from build123d import *

# Parameters (mm, degrees)
BASE_W                        = 80
BASE_H                        = 70
BASE_PLATE_DEPTH              = 3
EXTRUDER_HOLE_CUT_REACH       = 55.235
EXTRUDER_HOLE_R               = 20
EXTRUDER_SREW_HOLES_CUT_REACH = 55.235
EXTRUDER_MOUNT_HOLES_R        = 2.1
LM8_TWO_REACH                 = 55.235
LM8UU_HOLES_R                 = 1.7
LM8_CENTER_REACH              = 55.235
LM8UU_CENTER_R                = 1.7


with BuildPart() as part:
    # Base → Base Plate (new body)
    with BuildSketch(Plane(origin=(0, 0, 0), x_dir=(1, 0, 0), z_dir=(0, 1, 0))):
        Rectangle(BASE_W, BASE_H)
    extrude(amount=BASE_PLATE_DEPTH)

    # Extruder hole → Extruder Hole Cut (cut, up to next)
    with BuildSketch(Plane(origin=(0, 3, 0), x_dir=(1, 0, 0), z_dir=(0, 1, 0)), mode=Mode.PRIVATE) as extruder_hole_cut_sk1:
        with Locations(Location((0, 0, 0), (0, 0, 270))):
            Circle(EXTRUDER_HOLE_R)
    extruder_hole_cut_tool1 = extrude(extruder_hole_cut_sk1.sketch, amount=-EXTRUDER_HOLE_CUT_REACH, mode=Mode.PRIVATE) & part.part
    add(extruder_hole_cut_tool1.solids().sort_by_distance((0, 3, 0))[0], mode=Mode.SUBTRACT)

    # Extruder Mount Holes → Extruder Srew Holes Cut (cut, up to next)
    with BuildSketch(Plane(origin=(0, 3, 0), x_dir=(1, 0, 0), z_dir=(0, 1, 0)), mode=Mode.PRIVATE) as extruder_srew_holes_cut_sk1:
        with Locations(Location((-25, 0, 0), (0, 0, 270))):
            Circle(EXTRUDER_MOUNT_HOLES_R)
    extruder_srew_holes_cut_tool1 = extrude(extruder_srew_holes_cut_sk1.sketch, amount=-EXTRUDER_SREW_HOLES_CUT_REACH, mode=Mode.PRIVATE) & part.part
    # Extruder Mount Holes → Extruder Srew Holes Cut (cut, up to next)
    with BuildSketch(Plane(origin=(0, 3, 0), x_dir=(1, 0, 0), z_dir=(0, 1, 0)), mode=Mode.PRIVATE) as extruder_srew_holes_cut_sk2:
        with Locations(Location((-22.912878475, 10, 0), (0, 0, 270))):
            Circle(EXTRUDER_MOUNT_HOLES_R)
    extruder_srew_holes_cut_tool2 = extrude(extruder_srew_holes_cut_sk2.sketch, amount=-EXTRUDER_SREW_HOLES_CUT_REACH, mode=Mode.PRIVATE) & part.part
    # Extruder Mount Holes → Extruder Srew Holes Cut (cut, up to next)
    with BuildSketch(Plane(origin=(0, 3, 0), x_dir=(1, 0, 0), z_dir=(0, 1, 0)), mode=Mode.PRIVATE) as extruder_srew_holes_cut_sk3:
        with Locations(Location((-22.912878475, -10, 0), (0, 0, 270))):
            Circle(EXTRUDER_MOUNT_HOLES_R)
    extruder_srew_holes_cut_tool3 = extrude(extruder_srew_holes_cut_sk3.sketch, amount=-EXTRUDER_SREW_HOLES_CUT_REACH, mode=Mode.PRIVATE) & part.part
    # Extruder Mount Holes → Extruder Srew Holes Cut (cut, up to next)
    with BuildSketch(Plane(origin=(0, 3, 0), x_dir=(1, 0, 0), z_dir=(0, 1, 0)), mode=Mode.PRIVATE) as extruder_srew_holes_cut_sk4:
        with Locations(Location((25, 0, 0), (0, 0, 270))):
            Circle(EXTRUDER_MOUNT_HOLES_R)
    extruder_srew_holes_cut_tool4 = extrude(extruder_srew_holes_cut_sk4.sketch, amount=-EXTRUDER_SREW_HOLES_CUT_REACH, mode=Mode.PRIVATE) & part.part
    # Extruder Mount Holes → Extruder Srew Holes Cut (cut, up to next)
    with BuildSketch(Plane(origin=(0, 3, 0), x_dir=(1, 0, 0), z_dir=(0, 1, 0)), mode=Mode.PRIVATE) as extruder_srew_holes_cut_sk5:
        with Locations(Location((23, 9.797958971, 0), (0, 0, 270))):
            Circle(EXTRUDER_MOUNT_HOLES_R)
    extruder_srew_holes_cut_tool5 = extrude(extruder_srew_holes_cut_sk5.sketch, amount=-EXTRUDER_SREW_HOLES_CUT_REACH, mode=Mode.PRIVATE) & part.part
    # Extruder Mount Holes → Extruder Srew Holes Cut (cut, up to next)
    with BuildSketch(Plane(origin=(0, 3, 0), x_dir=(1, 0, 0), z_dir=(0, 1, 0)), mode=Mode.PRIVATE) as extruder_srew_holes_cut_sk6:
        with Locations(Location((23, -9.797958971, 0), (0, 0, 270))):
            Circle(EXTRUDER_MOUNT_HOLES_R)
    extruder_srew_holes_cut_tool6 = extrude(extruder_srew_holes_cut_sk6.sketch, amount=-EXTRUDER_SREW_HOLES_CUT_REACH, mode=Mode.PRIVATE) & part.part
    add(extruder_srew_holes_cut_tool1.solids().sort_by_distance((-25, 3, 0))[0], mode=Mode.SUBTRACT)
    add(extruder_srew_holes_cut_tool2.solids().sort_by_distance((-22.912878, 3, -10))[0], mode=Mode.SUBTRACT)
    add(extruder_srew_holes_cut_tool3.solids().sort_by_distance((-22.912878, 3, 10))[0], mode=Mode.SUBTRACT)
    add(extruder_srew_holes_cut_tool4.solids().sort_by_distance((25, 3, 0))[0], mode=Mode.SUBTRACT)
    add(extruder_srew_holes_cut_tool5.solids().sort_by_distance((23, 3, -9.797959))[0], mode=Mode.SUBTRACT)
    add(extruder_srew_holes_cut_tool6.solids().sort_by_distance((23, 3, 9.797959))[0], mode=Mode.SUBTRACT)

    # LM8uu Holes → LM8 Two (cut, up to next)
    with BuildSketch(Plane(origin=(0, 3, 0), x_dir=(1, 0, 0), z_dir=(0, 1, 0)), mode=Mode.PRIVATE) as lm8_two_sk1:
        with Locations(Location((-34, 29, 0), (0, 0, 270))):
            Circle(LM8UU_HOLES_R)
    lm8_two_tool1 = extrude(lm8_two_sk1.sketch, amount=-LM8_TWO_REACH, mode=Mode.PRIVATE) & part.part
    # LM8uu Holes → LM8 Two (cut, up to next)
    with BuildSketch(Plane(origin=(0, 3, 0), x_dir=(1, 0, 0), z_dir=(0, 1, 0)), mode=Mode.PRIVATE) as lm8_two_sk2:
        with Locations(Location((-28, 29, 0), (0, 0, 270))):
            Circle(LM8UU_HOLES_R)
    lm8_two_tool2 = extrude(lm8_two_sk2.sketch, amount=-LM8_TWO_REACH, mode=Mode.PRIVATE) & part.part
    # LM8uu Holes → LM8 Two (cut, up to next)
    with BuildSketch(Plane(origin=(0, 3, 0), x_dir=(1, 0, 0), z_dir=(0, 1, 0)), mode=Mode.PRIVATE) as lm8_two_sk3:
        with Locations(Location((28, 29, 0), (0, 0, 270))):
            Circle(LM8UU_HOLES_R)
    lm8_two_tool3 = extrude(lm8_two_sk3.sketch, amount=-LM8_TWO_REACH, mode=Mode.PRIVATE) & part.part
    # LM8uu Holes → LM8 Two (cut, up to next)
    with BuildSketch(Plane(origin=(0, 3, 0), x_dir=(1, 0, 0), z_dir=(0, 1, 0)), mode=Mode.PRIVATE) as lm8_two_sk4:
        with Locations(Location((34, 29, 0), (0, 0, 270))):
            Circle(LM8UU_HOLES_R)
    lm8_two_tool4 = extrude(lm8_two_sk4.sketch, amount=-LM8_TWO_REACH, mode=Mode.PRIVATE) & part.part
    add(lm8_two_tool1.solids().sort_by_distance((-34, 3, -29))[0], mode=Mode.SUBTRACT)
    add(lm8_two_tool2.solids().sort_by_distance((-28, 3, -29))[0], mode=Mode.SUBTRACT)
    add(lm8_two_tool3.solids().sort_by_distance((28, 3, -29))[0], mode=Mode.SUBTRACT)
    add(lm8_two_tool4.solids().sort_by_distance((34, 3, -29))[0], mode=Mode.SUBTRACT)

    # LM8uu Center → LM8 Center (cut, up to next)
    with BuildSketch(Plane(origin=(0, 3, 0), x_dir=(1, 0, 0), z_dir=(0, 1, 0)), mode=Mode.PRIVATE) as lm8_center_sk1:
        with Locations(Location((-3, -29, 0), (0, 0, 270))):
            Circle(LM8UU_CENTER_R)
    lm8_center_tool1 = extrude(lm8_center_sk1.sketch, amount=-LM8_CENTER_REACH, mode=Mode.PRIVATE) & part.part
    # LM8uu Center → LM8 Center (cut, up to next)
    with BuildSketch(Plane(origin=(0, 3, 0), x_dir=(1, 0, 0), z_dir=(0, 1, 0)), mode=Mode.PRIVATE) as lm8_center_sk2:
        with Locations(Location((3, -29, 0), (0, 0, 270))):
            Circle(LM8UU_CENTER_R)
    lm8_center_tool2 = extrude(lm8_center_sk2.sketch, amount=-LM8_CENTER_REACH, mode=Mode.PRIVATE) & part.part
    add(lm8_center_tool1.solids().sort_by_distance((-3, 3, 29))[0], mode=Mode.SUBTRACT)
    add(lm8_center_tool2.solids().sort_by_distance((3, 3, 29))[0], mode=Mode.SUBTRACT)


solid = part.part
CAD build for the part. Positions are in the model's coordinates, mm. Round coordinates to 2 decimals unless told otherwise and drop trailing zeros. Order: outer loops, then holes, each group sorted by start corner. A loop starts at its lowest first (then second) coordinate and runs counter-clockwise, first axis right, second up. Notation, with made-up numbers: (47, 51.25) -> (69, 51.25) arc R23 cw to (69, 66.25) -> close; hole circle Ø4 at (-35.75, 36.5). An arc over 180 degrees is marked (long way). Write item = value, one per line. Start each with the question number.
(1) Cut at B-B, the plane x = 28. List the corners of the cut face in (y, z), then the cut area to 3 significant figures.
(2) Cut at C-C, the plane z = 29. List the corners of the cut face in (x, y).
(3) Pull direction Z, two halves, no side cores. Call faces 1 (the flat face through (-18, 3, -16)), 2 (the cylindrical face through (-27.49, 1.52, -27.38)), 3 (the flat face through (-1, 1, 35)), 4 (the flat face through (-1, 1, -35)): released by +Z, released by -Z, zero draft, split by the parting line, or undercut.
(4) Cut at A-A, the plane z = 0. List the corners of the cut face in (x, y).
(5) Cut at D-D, the plane x = -3. List the corners of the cut face in (y, z), then the cut area to 3 significant figures.
(6) Probe line 1 (X direction, y = 1.65, z = 0); line 2 (X direction, y = 1.75, z = -10); line 3 (X direction, y = 1.2, z = 30). List the from-to ranges inside material, lowest first. Write a range as [from, to].
(7) Pin check, flat tip, straight feed: P1, Ø4, axis at x = -22.91, z = 10, coming from the +Y side. Stop position of the tip, or through.
Model answer:
q1.outline = (0, -35) -> (3, -35) -> (3, -30.7) -> (0, -30.7) -> close; (0, -27.3) -> (3, -27.3) -> (3, 35) -> (0, 35) -> close
q1.area = 200 mm2
q2.outline = (-40, 0) -> (-4.7, 0) -> (-4.7, 3) -> (-40, 3) -> close; (-1.3, 0) -> (1.3, 0) -> (1.3, 3) -> (-1.3, 3) -> close; (4.7, 0) -> (40, 0) -> (40, 3) -> (4.7, 3) -> close
q3.face_1 = zero draft
q3.face_2 = undercut
q3.face_3 = released by +Z
q3.face_4 = released by -Z
q4.outline = (-40, 0) -> (-27.1, 0) -> (-27.1, 3) -> (-40, 3) -> close; (-22.9, 0) -> (-20, 0) -> (-20, 3) -> (-22.9, 3) -> close; (20, 0) -> (22.9, 0) -> (22.9, 3) -> (20, 3) -> close; (27.1, 0) -> (40, 0) -> (40, 3) -> (27.1, 3) -> close
q5.outline = (0, -35) -> (3, -35) -> (3, -19.77) -> (0, -19.77) -> close; (0, 19.77) -> (3, 19.77) -> (3, 27.3) -> (0, 27.3) -> close; (0, 30.7) -> (3, 30.7) -> (3, 35) -> (0, 35) -> close
q5.area = 81.2 mm2
q6.line_1 = [-40, -27.1], [-22.9, -20], [20, 22.9], [27.1, 40]
q6.line_2 = [-40, -25.01], [-20.81, -17.32], [17.32, 20.91], [25.09, 40]
q6.line_3 = [-40, -4.37], [-1.63, 1.63], [4.37, 40]
q7.P1 = through
